Source: CAD feature listing. Evaluate the final solid. Frame: model axes, mm. Face numbers are marked on the shaded views. Give positions to 0.01 mm unless a question says otherwise; leave off trailing zeros. Loops run counter-clockwise (first coordinate to the right, second up) from the corner with the lowest first, then second, coordinate; pieces in that order, holes last. Notation, with made-up numbers: (-35.5, 63) - (23.5, 63) arc R37 ccw to (23.5, 99) - close; hole circle Ø11 at (18, -6.5). An arc over 180 degrees is marked (long way). Put each result on its own line as item: value.
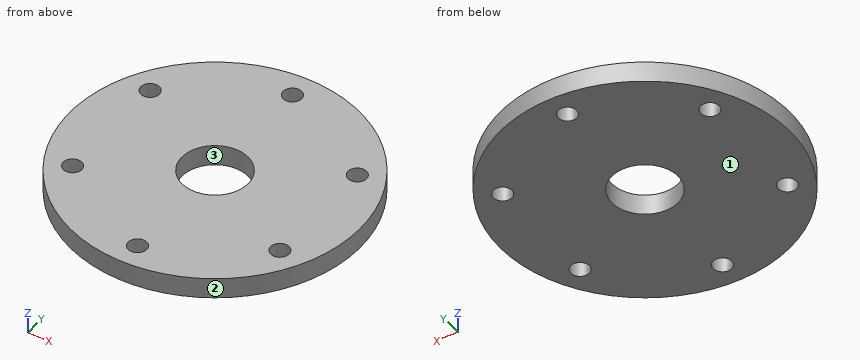
```python
from build123d import *

# Parameters (mm, degrees)
F0_R     = 35
F0_R_2   = 2.25
F0_R_3   = 8
F1_DEPTH = 5


with BuildPart() as f1:
    # F0 (on Top) → F1 (new body)
    with BuildSketch(Plane.XY):
        Circle(F0_R)
        with Locations((-25.114737, -14.5)):
            Circle(F0_R_2, mode=Mode.SUBTRACT)
        with Locations((0, -29)):
            Circle(F0_R_2, mode=Mode.SUBTRACT)
        with Locations((25.114737, -14.5)):
            Circle(F0_R_2, mode=Mode.SUBTRACT)
        with Locations((-25.114737, 14.5)):
            Circle(F0_R_2, mode=Mode.SUBTRACT)
        Circle(F0_R_3, mode=Mode.SUBTRACT)
        with Locations((25.114737, 14.5)):
            Circle(F0_R_2, mode=Mode.SUBTRACT)
        with Locations((0, 29)):
            Circle(F0_R_2, mode=Mode.SUBTRACT)
    extrude(amount=F1_DEPTH)


solid = f1.part
```
1) Section query D-D, the plane y = -13.5. Output: boundary loops of the cut face in (x, z), plus the area to 3 significant figures.
Check result:
outline: (-32.29, 0) - (-27.13, 0) - (-27.13, 5) - (-32.29, 5) - close; (-23.1, 0) - (23.1, 0) - (23.1, 5) - (-23.1, 5) - close; (27.13, 0) - (32.29, 0) - (32.29, 5) - (27.13, 5) - close
area: 283 mm²
2) Mould query, pull axis Y, two halves, no side actions, for the marked faces 1, 2 and 3. Classes: pulls with the +Y half, pulls with the -Y half, needs draft (parallel to the pull), parting line crosses it, or undercut.
Check result:
face 1: needs draft
face 2: parting line crosses it
face 3: undercut
3) Section query A-A, the plane y = 0. Output: boundary loops of the cut face in (x, z).
Check result:
outline: (-35, 0) - (-8, 0) - (-8, 5) - (-35, 5) - close; (8, 0) - (35, 0) - (35, 5) - (8, 5) - close
4) Material intervals for line 1 along Y through (x, z) = (0, 2.6); line 2 along X through (y, z) = (-0.5, 1); line 3 along X through (y, z) = (-15, 3.7), sorted ascending. Write a range as [from, to].
Check result:
line 1: [-35, -31.25], [-26.75, -8], [8, 26.75], [31.25, 35]
line 2: [-35, -7.98], [7.98, 35]
line 3: [-31.62, -27.31], [-22.92, 22.92], [27.31, 31.62]
5) Section query B-B, the plane x = 0. Output: boundary loops of the cut face in (y, z), plus the area to 3 significant figures.
Check result:
outline: (-35, 0) - (-31.25, 0) - (-31.25, 5) - (-35, 5) - close; (-26.75, 0) - (-8, 0) - (-8, 5) - (-26.75, 5) - close; (8, 0) - (26.75, 0) - (26.75, 5) - (8, 5) - close; (31.25, 0) - (35, 0) - (35, 5) - (31.25, 5) - close
area: 225 mm²
6) Section query C-C, the plane z = 2.4. Output: boundary loops of the cut face in (x, y), plus the area to 3 significant figures.
Check result:
outline: circle Ø70 at (0, 0); hole circle Ø4.5 at (-25.11, -14.5); hole circle Ø4.5 at (-25.11, 14.5); hole circle Ø16 at (0, 0); hole circle Ø4.5 at (0, -29); hole circle Ø4.5 at (0, 29); hole circle Ø4.5 at (25.11, -14.5); hole circle Ø4.5 at (25.11, 14.5)
area: 3,550 mm²
7) Pin query (flat end, axial travel): P1, Ø4, axis at x = 25.11, y = 14.5, coming from the -Z side; P2, Ø1.5, axis at x = 10, z = 2, coming from the +Y side; P3, Ø1.5, axis at y = -1, z = 2, coming from the -X side. Return the tip coordinate at first contact, or that it passes through.
Check result:
P1: through
P2: y = 33.76
P3: x = -35
